Answer from the drawing. Dimensions are ordinates in mm from the lowest x, y and z of the part. A direction names the side the tool comes from. Coordinates: 2 decimals unless noted, no trailing zeros. Loops run counter-clockwise (first coordinate to the right, second up) from the corner with the lowest first, then second, coordinate; pieces in that order, holes last.
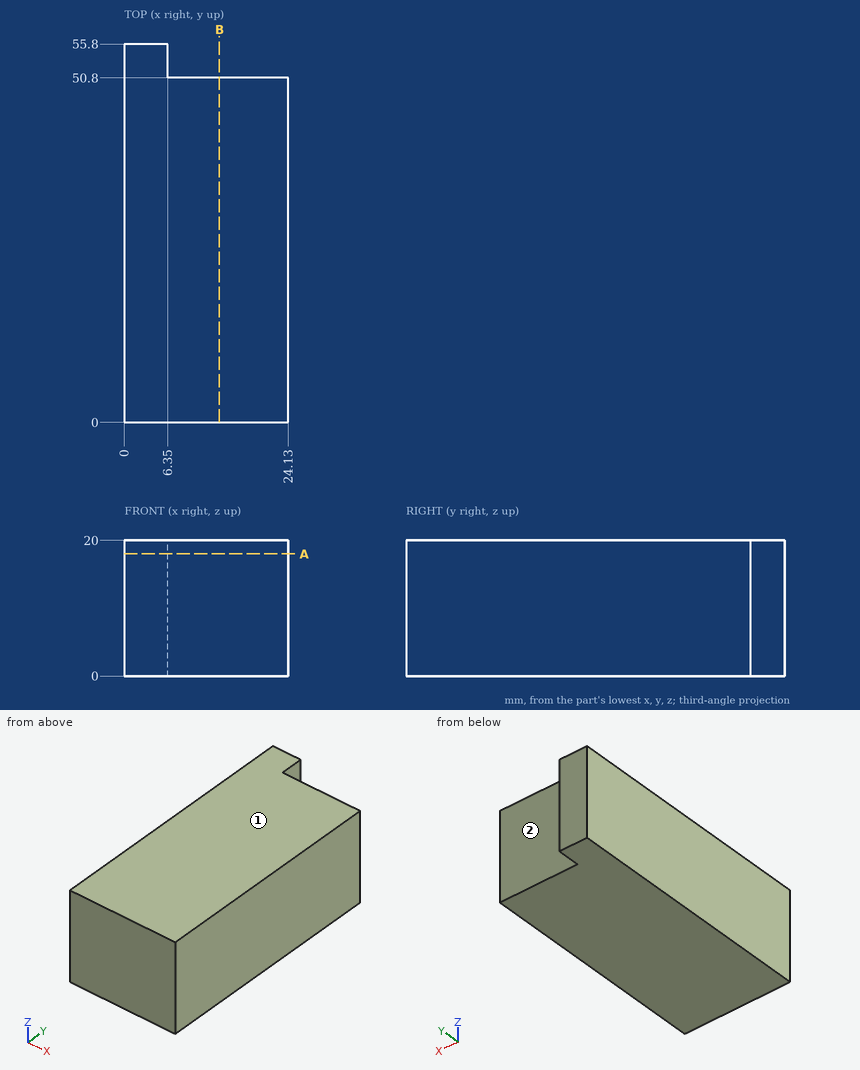
Item 1: A cutting plane is placed at B-B on x = 14. Determine the outline of the cut face in (y, z), then the cut area to 3 significant figures.
Numbers:
outline: (0, 0) - (50.8, 0) - (50.8, 20) - (0, 20) - close
area: 1,020 mm2
Item 2: A cutting plane is placed at A-A on z = 18. Determine the outline of the cut face in (x, y), then the cut area to 3 significant figures.
Numbers:
outline: (0, 0) - (24.13, 0) - (24.13, 50.8) - (6.35, 50.8) - (6.35, 55.8) - (0, 55.8) - close
area: 1,260 mm2
Item 3: Which of the six approach directions +Z, -Z, +X, -X, +Y, -Y give full straight-line access (tool end or side, diameter ignored) to the marked faces 1 and 2?
Numbers:
face 1: +Z, +X, -X, +Y, -Y
face 2: +Z, -Z, +X, +Y
Item 4: Given pin 1 (1.5 mm diameter, centred on y = 54, z = 12, fed in from +X); pin 2 (5 mm diameter, centred on x = 20.5, z = 3.5, fed in from +Y), each flat-ended and moving along its own axis, determine where each tip first touches the part or whether it passes through.
Numbers:
pin 1: stops at x = 6.35
pin 2: stops at y = 50.8
Item 5: Find the intervals of material crossed by line 1 along Y through (x, z) = (17, 18.75), in increasing order.
Numbers:
line 1: y = 0 to 50.8
